from build123d import *

# Parameters (mm, degrees)
F1_DEPTH = 10
F3_DEPTH = 5
F4_D     = 3


with BuildPart() as f1:
    # F0 (on Right) → F1 (new body, symmetric)
    with BuildSketch(Plane.YZ):
        with BuildLine():
            ThreePointArc((12, 0), (0, -12), (-12, 0))
            Line((-12, 0), (-17.0000008196, 0))
            ThreePointArc((-17.0000008196, 0), (-6.5192030966, -15.7003190684), (12, -12.0415957358))
            Line((12, -12.0415957358), (12, 0))
        make_face()
        with BuildLine():
            Line((17.0000008196, -30), (17.0000008196, 0))
            ThreePointArc((17.0000008196, 0), (15.7003190684, -6.5192030966), (12, -12.0415957358))
            Line((12, -12.0415957358), (12, -30))
            Line((12, -30), (17.0000008196, -30))
        make_face()
        with BuildLine():
            Line((17.0000008196, 0), (12, 0))
            Line((12, 0), (12, -12.0415957358))
            ThreePointArc((12, -12.0415957358), (15.7003190684, -6.5192030966), (17.0000008196, 0))
        make_face()
    extrude(amount=F1_DEPTH, both=True)

    # F3 (add): a face of the model
    f3_faces = [f1.faces().sort_by_distance(p)[0] for p in [
        (0, 14.5000004098, -30),
    ]]
    extrude(f3_faces, amount=F3_DEPTH)

    # F4 (through all)
    with Locations(Plane.XZ.offset(-12)):
        with Locations((0, -30), (0, -21.0207978679)):
            Hole(F4_D / 2)


solid = f1.part
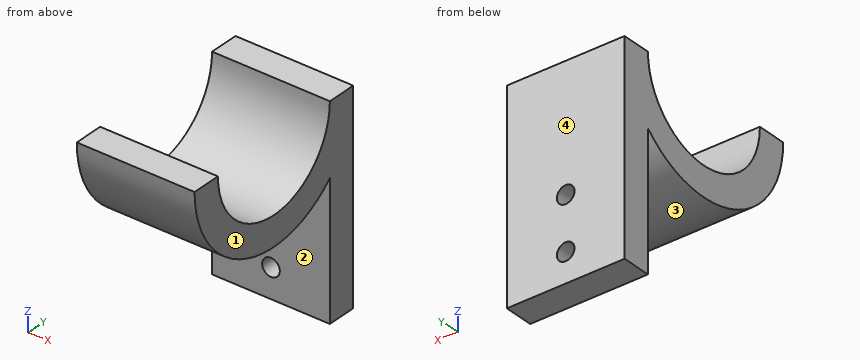
Here's how the part is built. I have some questions about the finished solid (model axes, mm). Face numbers are marked on the shaded views. Give positions to 0.01 mm unless a question says otherwise; leave off trailing zeros. Loops run counter-clockwise (first coordinate to the right, second up) from the corner with the lowest first, then second, coordinate; pieces in that order, holes last. Notation, with made-up numbers: (-6, 5) -> (44, 5) arc R14 ccw to (44, 31) -> close; hole circle Ø1 at (-23, -23). An arc over 180 degrees is marked (long way). Answer as a JSON object with one key per item and string values. Group by question number.
Item 1: Imagine slicing it at A-A on x = 0. Write out the boundary of the cut face in (y, z).
Item 2: Will these pins go through, and if not, where does the flat tip stop? pin 1 (3.5 mm diameter, centred on x = 0, z = -30, fed in from -Y); pin 2 (1 mm diameter, centred on x = -6.5, y = 4.5, fed in from -Z); pin 3 (1 mm diameter, centred on x = 1, z = -11, fed in from -Y).
Item 3: Thinking about a two-plate mould opening in Y: for the marked faces 1, 2, 3 and 4, which applies, pulls with the +Y half, pulls with the -Y half, needs draft (parallel to the pull), parting line crosses it, or undercut?
Item 4: I need wall thicknesses on L1, parallel to Z at x = 0, y = 13.3; L2, parallel to Y at x = -3.5, z = -2.5; L3, parallel to Y at x = -8.75, z = -25. Which ranges of each line are inside material? Lowest first, please.
Item 5: Imagine slicing it at C-C on x = -3.75. Write out the boundary of the cut face in (y, z), then the cut area to 3 significant figures.
Item 6: Imagine slicing it at D-D on y = 13.5. Write out the boundary of the cut face in (x, z), then the cut area to 3 significant figures.
Item 7: Imagine slicing it at B-B on z = -12.5. Write out the boundary of the cut face in (x, y).
Answer list:
{
 "1": {"outline": "(-17, 0) arc R17 ccw to (12, -12.04) -> (12, -19.52) -> (17, -19.52) -> (17, 0) -> (12, 0) arc R12 cw to (-12, 0) -> close; (12, -35) -> (17, -35) -> (17, -31.5) -> (12, -31.5) -> close; (12, -28.5) -> (17, -28.5) -> (17, -22.52) -> (12, -22.52) -> close"},
 "2": {"pin 1": "stops at y = 12", "pin 2": "stops at z = -16.52", "pin 3": "stops at y = -13.37"},
 "3": {"face 1": "needs draft", "face 2": "undercut", "face 3": "undercut", "face 4": "pulls with the +Y half"},
 "4": {"L1": "z = -35 to -31.5, -28.5 to -22.52, -19.52 to 0", "L2": "y = -16.82 to -11.74, 11.74 to 17", "L3": "y = 12 to 17"},
 "5": {"outline": "(-17, 0) arc R17 ccw to (12, -12.04) -> (12, -35) -> (17, -35) -> (17, 0) -> (12, 0) arc R12 cw to (-12, 0) -> close", "area": "361 mm2"},
 "6": {"outline": "(-10, -35) -> (10, -35) -> (10, 0) -> (-10, 0) -> close; hole circle Ø3 at (0, -30); hole circle Ø3 at (0, -21.02)", "area": "686 mm2"},
 "7": {"outline": "(-10, -11.52) -> (10, -11.52) -> (10, 11.52) -> (-10, 11.52) -> close; (-10, 12) -> (10, 12) -> (10, 17) -> (-10, 17) -> close"}
}
